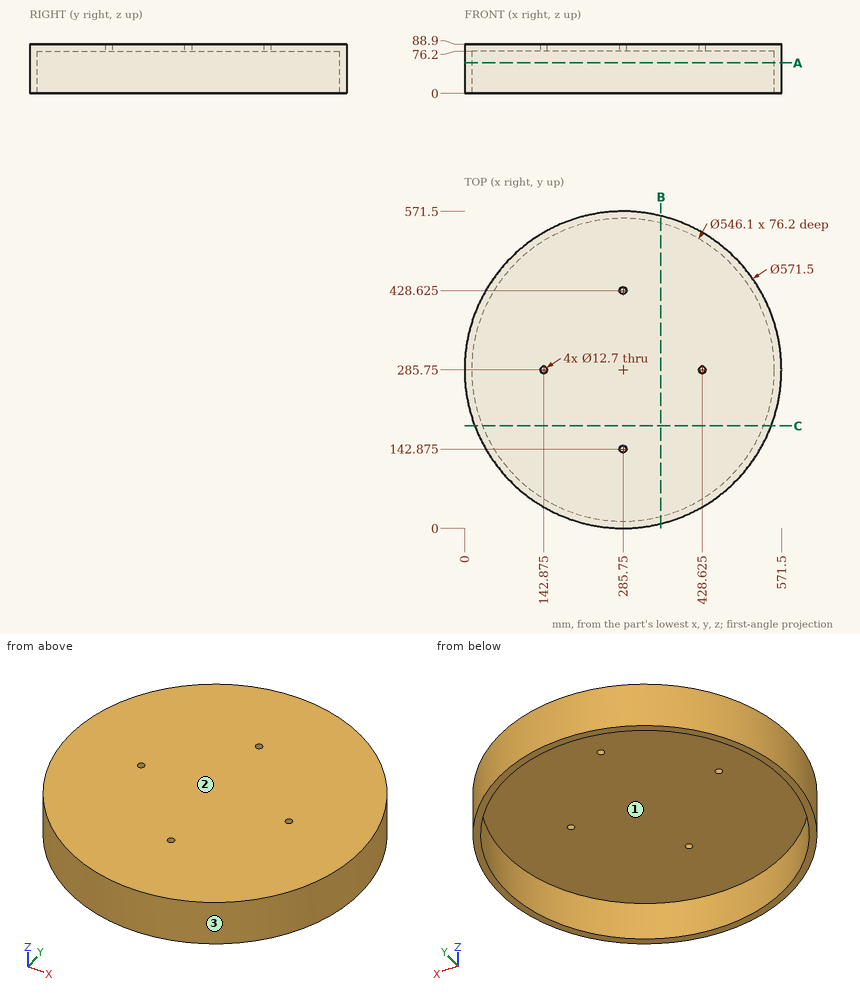
Geometry: see drawing. Coordinates: mm, zero at the bounding-box minimum. Coordinates: 2 decimals unless noted, no trailing zeros. Order: outer loops, then holes, each group sorted by start corner. A loop starts at its lowest first (then second) coordinate and runs counter-clockwise, first axis right, second up. Notation, with made-up numbers: (77.25, 25.5) - (110.25, 25.5) arc R14 ccw to (110.25, 31.5) - close; hole circle Ø3 at (-29, -1.75). An arc over 180 degrees is marked (long way). Write each question's results on one line, items separated by ' | '.
1) Pin query (flat end, axial travel): pin 1 (20.5 mm diameter, centred on x = 285.75, y = 428.625, fed in from -Z); pin 2 (1 mm diameter, centred on y = 489, z = 59, fed in from -X); pin 3 (5 mm diameter, centred on y = 161, z = 39.5, fed in from -X). Return the tip coordinate at first contact, or that it passes through.
Results list:
pin 1: z = 76.2 | pin 2: x = 84.39 | pin 3: x = 27.47
2) Pull-direction query (X, two-part tool) for the marked faces 1, 2 and 3; classes: pulls with the +X half, pulls with the -X half, needs draft (parallel to the pull), parting line crosses it, or undercut.
Results list:
face 1: undercut | face 2: needs draft | face 3: parting line crosses it
3) Section B-B, the plane x = 354. Return loops of the section in (y, z), plus the area to 3 significant figures.
Results list:
outline: (8.27, 0) - (21.37, 0) - (21.37, 76.2) - (550.13, 76.2) - (550.13, 0) - (563.23, 0) - (563.23, 88.9) - (8.27, 88.9) - close | area: 9,040 mm^2
4) Section C-C, the plane y = 184.5. Return loops of the section in (x, z).
Results list:
outline: (18.54, 0) - (32.17, 0) - (32.17, 76.2) - (539.33, 76.2) - (539.33, 0) - (552.96, 0) - (552.96, 88.9) - (18.54, 88.9) - close
5) Line query: line 1 (X direction, y = 285, z = 82); line 2 (X direction, y = 281, z = 20). Output: solid intervals per line, ascending. Write a range as from..to.
Results list:
line 1: 0..136.57, 149.18..422.32, 434.93..571.5 | line 2: 0.04..12.74, 558.76..571.46
6) Section A-A, the plane z = 55. Return loops of the section in (x, y), plus the area to 3 significant figures.
Results list:
outline: circle Ø571.5 at (285.75, 285.75); hole circle Ø546.1 at (285.75, 285.75) | area: 22,300 mm^2
